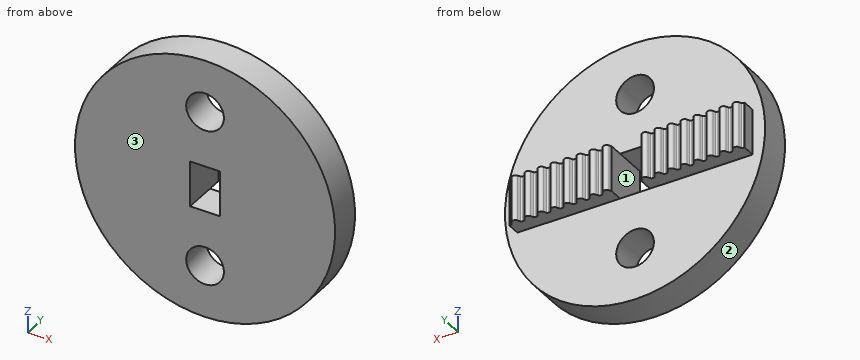
```python
from build123d import *

# Parameters (mm, degrees)
BOSS_EXTRUDE1_DEPTH     = 7
BOSS_EXTRUDE2_START     = -2
SKETCH2_R               = 20
BOSS_EXTRUDE2_DEPTH     = 5
CUT_EXTRUDE2_DEPTH      = 46.034410177
CUT_EXTRUDE2_DEPTH_BACK = 46.034410177
SKETCH4_W               = 4.6
SKETCH4_H               = 7
M5_CLEARANCE_HOLE1_D    = 5.8


with BuildPart() as part:
    # Sketch1 → Boss-Extrude1 (new body)
    with BuildSketch(Plane.XY):
        with BuildLine():
            Line((3.767777778, 0.135469288), (3.578888889, 0.501967566))
            ThreePointArc((3.578888889, 0.501967566), (3.09, 0.8), (2.601111111, 0.501967566))
            Line((2.601111111, 0.501967566), (2.412222222, 0.135469288))
            ThreePointArc((2.412222222, 0.135469288), (2.320129401, 0.036537266), (2.19, 0))
            Line((2.19, 0), (2.18, 0))
            Line((2.18, 0), (2, 0))
            Line((2, 0), (1.99, 0))
            ThreePointArc((1.99, 0), (1.859870599, 0.036537266), (1.767777778, 0.135469288))
            Line((1.767777778, 0.135469288), (1.578888889, 0.501967566))
            ThreePointArc((1.578888889, 0.501967566), (1.09, 0.8), (0.601111111, 0.501967566))
            Line((0.601111111, 0.501967566), (0.412222222, 0.135469288))
            ThreePointArc((0.412222222, 0.135469288), (0.320129401, 0.036537266), (0.19, 0))
            Line((0.19, 0), (0, 0))
            Line((0, 0), (0, -5))
            Line((0, -5), (36.18, -5))
            Line((36.18, -5), (36.18, 0))
            Line((36.18, 0), (35.99, 0))
            ThreePointArc((35.99, 0), (35.859870599, 0.036537266), (35.767777778, 0.135469288))
            Line((35.767777778, 0.135469288), (35.578888889, 0.501967566))
            ThreePointArc((35.578888889, 0.501967566), (35.09, 0.8), (34.601111111, 0.501967566))
            Line((34.601111111, 0.501967566), (34.412222222, 0.135469288))
            ThreePointArc((34.412222222, 0.135469288), (34.320129401, 0.036537266), (34.19, 0))
            Line((34.19, 0), (34.18, 0))
            Line((34.18, 0), (34, 0))
            Line((34, 0), (33.99, 0))
            ThreePointArc((33.99, 0), (33.859870599, 0.036537266), (33.767777778, 0.135469288))
            Line((33.767777778, 0.135469288), (33.578888889, 0.501967566))
            ThreePointArc((33.578888889, 0.501967566), (33.09, 0.8), (32.601111111, 0.501967566))
            Line((32.601111111, 0.501967566), (32.412222222, 0.135469288))
            ThreePointArc((32.412222222, 0.135469288), (32.320129401, 0.036537266), (32.19, 0))
            Line((32.19, 0), (32.18, 0))
            Line((32.18, 0), (32, 0))
            Line((32, 0), (31.99, 0))
            ThreePointArc((31.99, 0), (31.859870599, 0.036537266), (31.767777778, 0.135469288))
            Line((31.767777778, 0.135469288), (31.578888889, 0.501967566))
            ThreePointArc((31.578888889, 0.501967566), (31.09, 0.8), (30.601111111, 0.501967566))
            Line((30.601111111, 0.501967566), (30.412222222, 0.135469288))
            ThreePointArc((30.412222222, 0.135469288), (30.320129401, 0.036537266), (30.19, 0))
            Line((30.19, 0), (30.18, 0))
            Line((30.18, 0), (30, 0))
            Line((30, 0), (29.99, 0))
            ThreePointArc((29.99, 0), (29.859870599, 0.036537266), (29.767777778, 0.135469288))
            Line((29.767777778, 0.135469288), (29.578888889, 0.501967566))
            ThreePointArc((29.578888889, 0.501967566), (29.09, 0.8), (28.601111111, 0.501967566))
            Line((28.601111111, 0.501967566), (28.412222222, 0.135469288))
            ThreePointArc((28.412222222, 0.135469288), (28.320129401, 0.036537266), (28.19, 0))
            Line((28.19, 0), (28.18, 0))
            Line((28.18, 0), (28, 0))
            Line((28, 0), (27.99, 0))
            ThreePointArc((27.99, 0), (27.859870599, 0.036537266), (27.767777778, 0.135469288))
            Line((27.767777778, 0.135469288), (27.578888889, 0.501967566))
            ThreePointArc((27.578888889, 0.501967566), (27.09, 0.8), (26.601111111, 0.501967566))
            Line((26.601111111, 0.501967566), (26.412222222, 0.135469288))
            ThreePointArc((26.412222222, 0.135469288), (26.320129401, 0.036537266), (26.19, 0))
            Line((26.19, 0), (26.18, 0))
            Line((26.18, 0), (26, 0))
            Line((26, 0), (25.99, 0))
            ThreePointArc((25.99, 0), (25.859870599, 0.036537266), (25.767777778, 0.135469288))
            Line((25.767777778, 0.135469288), (25.578888889, 0.501967566))
            ThreePointArc((25.578888889, 0.501967566), (25.09, 0.8), (24.601111111, 0.501967566))
            Line((24.601111111, 0.501967566), (24.412222222, 0.135469288))
            ThreePointArc((24.412222222, 0.135469288), (24.320129401, 0.036537266), (24.19, 0))
            Line((24.19, 0), (24.18, 0))
            Line((24.18, 0), (24, 0))
            Line((24, 0), (23.99, 0))
            ThreePointArc((23.99, 0), (23.859870599, 0.036537266), (23.767777778, 0.135469288))
            Line((23.767777778, 0.135469288), (23.578888889, 0.501967566))
            ThreePointArc((23.578888889, 0.501967566), (23.09, 0.8), (22.601111111, 0.501967566))
            Line((22.601111111, 0.501967566), (22.412222222, 0.135469288))
            ThreePointArc((22.412222222, 0.135469288), (22.320129401, 0.036537266), (22.19, 0))
            Line((22.19, 0), (22.18, 0))
            Line((22.18, 0), (22, 0))
            Line((22, 0), (21.99, 0))
            ThreePointArc((21.99, 0), (21.859870599, 0.036537266), (21.767777778, 0.135469288))
            Line((21.767777778, 0.135469288), (21.578888889, 0.501967566))
            ThreePointArc((21.578888889, 0.501967566), (21.09, 0.8), (20.601111111, 0.501967566))
            Line((20.601111111, 0.501967566), (20.412222222, 0.135469288))
            ThreePointArc((20.412222222, 0.135469288), (20.320129401, 0.036537266), (20.19, 0))
            Line((20.19, 0), (20.18, 0))
            Line((20.18, 0), (20, 0))
            Line((20, 0), (19.99, 0))
            ThreePointArc((19.99, 0), (19.859870599, 0.036537266), (19.767777778, 0.135469288))
            Line((19.767777778, 0.135469288), (19.578888889, 0.501967566))
            ThreePointArc((19.578888889, 0.501967566), (19.09, 0.8), (18.601111111, 0.501967566))
            Line((18.601111111, 0.501967566), (18.412222222, 0.135469288))
            ThreePointArc((18.412222222, 0.135469288), (18.320129401, 0.036537266), (18.19, 0))
            Line((18.19, 0), (18.18, 0))
            Line((18.18, 0), (18, 0))
            Line((18, 0), (17.99, 0))
            ThreePointArc((17.99, 0), (17.859870599, 0.036537266), (17.767777778, 0.135469288))
            Line((17.767777778, 0.135469288), (17.578888889, 0.501967566))
            ThreePointArc((17.578888889, 0.501967566), (17.09, 0.8), (16.601111111, 0.501967566))
            Line((16.601111111, 0.501967566), (16.412222222, 0.135469288))
            ThreePointArc((16.412222222, 0.135469288), (16.320129401, 0.036537266), (16.19, 0))
            Line((16.19, 0), (16.18, 0))
            Line((16.18, 0), (16, 0))
            Line((16, 0), (15.99, 0))
            ThreePointArc((15.99, 0), (15.859870599, 0.036537266), (15.767777778, 0.135469288))
            Line((15.767777778, 0.135469288), (15.578888889, 0.501967566))
            ThreePointArc((15.578888889, 0.501967566), (15.09, 0.8), (14.601111111, 0.501967566))
            Line((14.601111111, 0.501967566), (14.412222222, 0.135469288))
            ThreePointArc((14.412222222, 0.135469288), (14.320129401, 0.036537266), (14.19, 0))
            Line((14.19, 0), (14.18, 0))
            Line((14.18, 0), (14, 0))
            Line((14, 0), (13.99, 0))
            ThreePointArc((13.99, 0), (13.859870599, 0.036537266), (13.767777778, 0.135469288))
            Line((13.767777778, 0.135469288), (13.578888889, 0.501967566))
            ThreePointArc((13.578888889, 0.501967566), (13.09, 0.8), (12.601111111, 0.501967566))
            Line((12.601111111, 0.501967566), (12.412222222, 0.135469288))
            ThreePointArc((12.412222222, 0.135469288), (12.320129401, 0.036537266), (12.19, 0))
            Line((12.19, 0), (12.18, 0))
            Line((12.18, 0), (12, 0))
            Line((12, 0), (11.99, 0))
            ThreePointArc((11.99, 0), (11.859870599, 0.036537266), (11.767777778, 0.135469288))
            Line((11.767777778, 0.135469288), (11.578888889, 0.501967566))
            ThreePointArc((11.578888889, 0.501967566), (11.09, 0.8), (10.601111111, 0.501967566))
            Line((10.601111111, 0.501967566), (10.412222222, 0.135469288))
            ThreePointArc((10.412222222, 0.135469288), (10.320129401, 0.036537266), (10.19, 0))
            Line((10.19, 0), (10.18, 0))
            Line((10.18, 0), (10, 0))
            Line((10, 0), (9.99, 0))
            ThreePointArc((9.99, 0), (9.859870599, 0.036537266), (9.767777778, 0.135469288))
            Line((9.767777778, 0.135469288), (9.578888889, 0.501967566))
            ThreePointArc((9.578888889, 0.501967566), (9.09, 0.8), (8.601111111, 0.501967566))
            Line((8.601111111, 0.501967566), (8.412222222, 0.135469288))
            ThreePointArc((8.412222222, 0.135469288), (8.320129401, 0.036537266), (8.19, 0))
            Line((8.19, 0), (8.18, 0))
            Line((8.18, 0), (8, 0))
            Line((8, 0), (7.99, 0))
            ThreePointArc((7.99, 0), (7.859870599, 0.036537266), (7.767777778, 0.135469288))
            Line((7.767777778, 0.135469288), (7.578888889, 0.501967566))
            ThreePointArc((7.578888889, 0.501967566), (7.09, 0.8), (6.601111111, 0.501967566))
            Line((6.601111111, 0.501967566), (6.412222222, 0.135469288))
            ThreePointArc((6.412222222, 0.135469288), (6.320129401, 0.036537266), (6.19, 0))
            Line((6.19, 0), (6.18, 0))
            Line((6.18, 0), (6, 0))
            Line((6, 0), (5.99, 0))
            ThreePointArc((5.99, 0), (5.859870599, 0.036537266), (5.767777778, 0.135469288))
            Line((5.767777778, 0.135469288), (5.578888889, 0.501967566))
            ThreePointArc((5.578888889, 0.501967566), (5.09, 0.8), (4.601111111, 0.501967566))
            Line((4.601111111, 0.501967566), (4.412222222, 0.135469288))
            ThreePointArc((4.412222222, 0.135469288), (4.320129401, 0.036537266), (4.19, 0))
            Line((4.19, 0), (4.18, 0))
            Line((4.18, 0), (4, 0))
            Line((4, 0), (3.99, 0))
            ThreePointArc((3.99, 0), (3.859870599, 0.036537266), (3.767777778, 0.135469288))
        make_face()
    extrude(amount=BOSS_EXTRUDE1_DEPTH)

    # Sketch2 → Boss-Extrude2 (add)
    with BuildSketch(Plane(origin=(0, 0, 0), x_dir=(1, 0, 0), z_dir=(0, 1, 0)).offset(BOSS_EXTRUDE2_START)):
        with Locations(Location((18.09, -3.5, 0), (0, 0, 270))):
            Circle(SKETCH2_R)
    extrude(amount=-BOSS_EXTRUDE2_DEPTH)

    # Sketch4 → Cut-Extrude2 (cut, two sides: drawn at the far end of the back side and taken through both)
    with BuildSketch(Plane(origin=(0, -2, 0), x_dir=(1, 0, 0), z_dir=(0, 1, 0)).offset(-CUT_EXTRUDE2_DEPTH_BACK)):
        with Locations((18.09, -3.5)):
            Rectangle(SKETCH4_W, SKETCH4_H)
    extrude(amount=CUT_EXTRUDE2_DEPTH + CUT_EXTRUDE2_DEPTH_BACK, mode=Mode.SUBTRACT)

    # M5 Clearance Hole1 (through all)
    with Locations(Plane(origin=(18.09, -7, 15.5), x_dir=(0, 0, -1), z_dir=(0, -1, 0))):
        with Locations((0, 0), (24, 0)):
            Hole(M5_CLEARANCE_HOLE1_D / 2)


solid = part.part
```
For this review, take the finished solid that the model builds, in its own axes (mm). Face numbers are marked on the shaded views. Coordinates: 2 decimals unless noted, no trailing zeros. Loops run counter-clockwise (first coordinate to the right, second up) from the corner with the lowest first, then second, coordinate; pieces in that order, holes last. Notation, with made-up numbers: (63, 43.25) -> (99, 43.25) arc R21 cw to (99, 63.25) -> close; hole circle Ø2 at (-30, 14). An arc over 180 degrees is marked (long way). Return JSON: item names as keys, results as strings. Group by question number.
(1) Consider section A-A, the plane y = -1.25. Give the boundary of the cut face in (x, z), plus the area to 3 significant figures.
(2) To check wall thickness, follow L1, parallel to Z at x = 18, y = -6.25; L2, parallel to X at y = -3.3, z = -8.5; L3, parallel to Z at x = 26.5, y = 0. State the ranges of each line that lie inside material, in increasing order.
(3) Mouldability with a two-part tool opening along X and no side actions: class the marked faces 1, 2 and 3 as pulls with the +X half, pulls with the -X half, needs draft (parallel to the pull), parting line crosses it, or undercut.
(4) For pin 1 Ø1.5 at (y, z) = (-4.5, -5) entering from +X; pin 2 Ø3 at (x, y) = (24.5, -4) entering from +Z; pin 3 Ø3 at (x, y) = (34, -3.5) entering from +Z, all flat-tipped, find the tip position at first contact; note any pin that passes through.
(5) Consider section B-B, the plane x = 18.09. Give the boundary of the cut face in (y, z), plus the area to 3 significant figures.
(6) Consider section C-C, the plane z = 15.5. Give the boundary of the cut face in (x, y).
(7) Consider section D-D, the plane y = -4.5. Give the boundary of the cut face in (x, z).
Results below:
{
 "1": {"outline": "(0, 0) -> (15.79, 0) -> (15.79, 7) -> (0, 7) -> close; (20.39, 0) -> (36.18, 0) -> (36.18, 7) -> (20.39, 7) -> close", "area": "221 mm2"},
 "2": {"L1": "z = -16.5 to -11.4, -5.6 to 0, 7 to 12.6, 18.4 to 23.5", "L2": "x = 2.09 to 15.19, 20.99 to 34.09", "L3": "z = 0 to 7"},
 "3": {"face 1": "undercut", "face 2": "parting line crosses it", "face 3": "needs draft"},
 "4": {"pin 1": "stops at x = 36.53", "pin 2": "stops at z = 22.89", "pin 3": "stops at z = 17.37"},
 "5": {"outline": "(-7, -16.5) -> (-2, -16.5) -> (-2, -11.4) -> (-7, -11.4) -> close; (-7, -5.6) -> (-2, -5.6) -> (-2, 0) -> (-7, 0) -> close; (-7, 7) -> (-2, 7) -> (-2, 12.6) -> (-7, 12.6) -> close; (-7, 18.4) -> (-2, 18.4) -> (-2, 23.5) -> (-7, 23.5) -> close", "area": "107 mm2"},
 "6": {"outline": "(2.09, -7) -> (15.19, -7) -> (15.19, -2) -> (2.09, -2) -> close; (20.99, -7) -> (34.09, -7) -> (34.09, -2) -> (20.99, -2) -> close"},
 "7": {"outline": "circle Ø40 at (18.09, 3.5); hole circle Ø5.8 at (18.09, -8.5); hole circle Ø5.8 at (18.09, 15.5); hole (15.79, 0) -> (20.39, 0) -> (20.39, 7) -> (15.79, 7) -> close"}
}
